Work out the finished part from the listing and answer in its coordinate system (mm). Coordinates: 2 decimals unless noted, no trailing zeros. Write each loop counter-clockwise with the first axis right and the second up, starting at its lowest first coordinate (ties: lowest second). Pieces come first, ordered by that corner, then holes. Notation, with made-up numbers: M -18.75,6 L -9.75,6 A7 ccw -9.75,18 Z; hole C 29.25,28 d5. An arc over 180 degrees is marked long. Use CSV: the item, a comma, the result in double quotes.
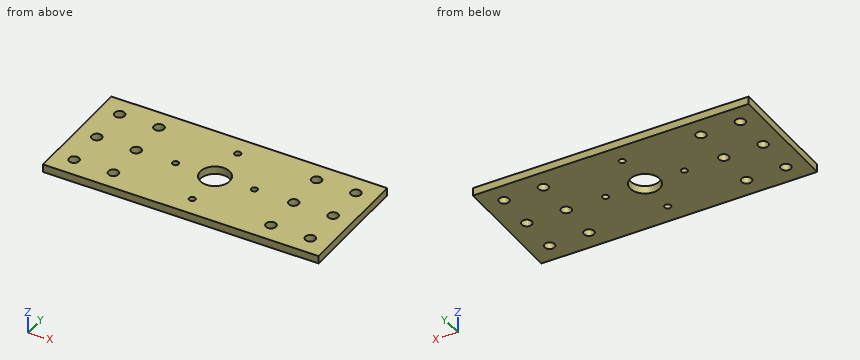
Autodesk Inventor part; units mm, degrees
ref_plane "YZ Plane" through (0, 0, 0) normal (1, 0, 0) x (0, 1, 0)
ref_plane "XZ Plane" through (0, 0, 0) normal (0, 1, 0) x (-1, 0, 0)
ref_plane "XY Plane" through (0, 0, 0) normal (0, 0, 1) x (1, 0, 0)
sketch "Sketch1" plane through (0, 0, 0) normal (0, 0, 1) x (1, 0, 0)
  line L0 (0, 0) -> (177.8, 0)
  line L1 (177.8, 0) -> (177.8, 76.2)
  line L2 (177.8, 76.2) -> (0, 76.2)
  line L3 (0, 76.2) -> (0, 0)
  circle A0 centre (88.9, 38.1) radius 9.525
  circle A1 centre (88.9, 63.5) radius 2.0193
  circle A2 centre (63.5, 38.1) radius 2.0193
  circle A3 centre (88.9, 12.7) radius 2.0193
  circle A4 centre (114.3, 38.1) radius 2.0193
  circle A5 centre (12.7, 63.5) radius 3.2512
  circle A6 centre (12.7, 38.1) radius 3.2512
  circle A7 centre (12.7, 12.7) radius 3.2512
  circle A8 centre (38.1, 63.5) radius 3.2512
  circle A9 centre (38.1, 38.1) radius 3.2512
  circle A10 centre (38.1, 12.7) radius 3.2512
  circle A11 centre (165.1, 63.5) radius 3.2512
  circle A12 centre (165.1, 38.1) radius 3.2512
  circle A13 centre (165.1, 12.7) radius 3.2512
  circle A14 centre (139.7, 63.5) radius 3.2512
  circle A15 centre (139.7, 38.1) radius 3.2512
  circle A16 centre (139.7, 12.7) radius 3.2512
  dimension "d0" = 177.8
  dimension "d1" = 76.2
  dimension "d2" = 19.05
  dimension "d3" = 38.1
  dimension "d4" = 88.9
  dimension "d5" = 4.0386
  dimension "d6" = 25.4
  dimension "d7" = 88.9
  dimension "d8" = 4.0386
  dimension "d9" = 25.4
  dimension "d10" = 38.1
  dimension "d13" = 50.8
  dimension "d20" = 50.8
  dimension "d25" = 6.5024
  dimension "d26" = 12.7
  dimension "d27" = 12.7
  dimension "d30" = 25.4
  dimension "d39" = 25.4
  dimension "d48" = 127
  dimension "d55" = 25.4
extrude "Extrusion3" add sketch "Sketch1" along normal blind 5.08
equation "\"d7\" = d4"
equation "\"d8\" = d5"
equation "\"d9\" = d6"
equation "\"d10\" = d3"
properties part number "Motor Mount Long"
Item 1: The part is cut by section D-D (x = 63.5). Write down the section's boundary in (y, z), then the cut area to 3 significant figures.
Answer:
outline,"M 0,0 L 36.08,0 L 36.08,5.08 L 0,5.08 Z; M 40.12,0 L 76.2,0 L 76.2,5.08 L 40.12,5.08 Z"
area,"367 mm2"
Item 2: The part is cut by section A-A (x = 165.1). Write down the section's boundary in (y, z), then the cut area to 3 significant figures.
Answer:
outline,"M 0,0 L 9.45,0 L 9.45,5.08 L 0,5.08 Z; M 15.95,0 L 34.85,0 L 34.85,5.08 L 15.95,5.08 Z; M 41.35,0 L 60.25,0 L 60.25,5.08 L 41.35,5.08 Z; M 66.75,0 L 76.2,0 L 76.2,5.08 L 66.75,5.08 Z"
area,"288 mm2"
Item 3: The part is cut by section C-C (y = 63.5). Write down the section's boundary in (x, z), then the cut area to 3 significant figures.
Answer:
outline,"M 0,0 L 9.45,0 L 9.45,5.08 L 0,5.08 Z; M 15.95,0 L 34.85,0 L 34.85,5.08 L 15.95,5.08 Z; M 41.35,0 L 86.88,0 L 86.88,5.08 L 41.35,5.08 Z; M 90.92,0 L 136.45,0 L 136.45,5.08 L 90.92,5.08 Z; M 142.95,0 L 161.85,0 L 161.85,5.08 L 142.95,5.08 Z; M 168.35,0 L 177.8,0 L 177.8,5.08 L 168.35,5.08 Z"
area,"751 mm2"
Item 4: The part is cut by section B-B (z = 2.7). Count the separate pieces of the cut face and the enclosed holes in it, then the cut area to 3 significant figures.
Answer:
separate pieces,"1"
enclosed holes,"17"
area,"12,800 mm2"
Item 5: Consider probe 1 along Y at (x, z) = (38.1, 3.45); probe 2 along X at (y, z) = (13, 3.2); probe 3 along X at (y, z) = (13.5, 3.8). Determine where each line is inside the solid, lowest interval first.
Answer:
probe 1,"y = 0 to 9.45, 15.95 to 34.85, 41.35 to 60.25, 66.75 to 76.2"
probe 2,"x = 0 to 9.46, 15.94 to 34.86, 41.34 to 86.9, 90.9 to 136.46, 142.94 to 161.86, 168.34 to 177.8"
probe 3,"x = 0 to 9.55, 15.85 to 34.95, 41.25 to 87.05, 90.75 to 136.55, 142.85 to 161.95, 168.25 to 177.8"
